from build123d import *

# Parameters (mm, degrees)
F1_DEPTH = 10.414
F2_W     = 50.8
F2_H     = 38.1
F2_R     = 17.78
F2_R_2   = 7.62
F3_DEPTH = 2.54
F4_W     = 10.16
F4_H     = 2.54
F4_R     = 1.27
F5_DEPTH = 5.08
F6_W     = 12.7
F6_H     = 2.54
F7_DEPTH = 5.08


with BuildPart() as f1:
    # F0 (on Front) → F1 (new body)
    with BuildSketch(Plane.XZ):
        with BuildLine():
            Line((-5.08, 57.662666), (-55.88, 57.662666))
            ThreePointArc((-55.88, 57.662666), (-59.472102, 56.174768), (-60.96, 52.582666))
            Line((-60.96, 52.582666), (-60.96, -41.397334))
            ThreePointArc((-60.96, -41.397334), (-59.472102, -44.989437), (-55.88, -46.477334))
            Line((-55.88, -46.477334), (-5.08, -46.477334))
            ThreePointArc((-5.08, -46.477334), (-1.487898, -44.989437), (0, -41.397334))
            Line((0, -41.397334), (0, 52.582666))
            ThreePointArc((0, 52.582666), (-1.487898, 56.174768), (-5.08, 57.662666))
        make_face()
    extrude(amount=F1_DEPTH)

    # F2 (on face) → F3 (join)
    with BuildSketch(Plane.XZ.offset(10.414)):
        with Locations((-30.48, 33.532666)):
            Rectangle(F2_W, F2_H)
        with Locations((-30.48, -15.997334)):
            Circle(F2_R)
        with Locations((-30.48, -15.997334)):
            Circle(F2_R_2, mode=Mode.SUBTRACT)
    extrude(amount=F3_DEPTH)

    # F4 (on face) → F5 (cut)
    with BuildSketch(Plane.XY.offset(57.662666)):
        with Locations((-48.26, -6.604)):
            Rectangle(F4_W, F4_H)
        with Locations((-9.593616, -6.604)):
            Circle(F4_R)
    extrude(amount=-F5_DEPTH, mode=Mode.SUBTRACT)

    # F6 (on face) → F7 (cut)
    with BuildSketch(Plane(origin=(0, 0, -46.477334), x_dir=(1, 0, 0), z_dir=(0, 0, -1))):
        with Locations((-30.48, 7.796658)):
            Rectangle(F6_W, F6_H)
    extrude(amount=-F7_DEPTH, mode=Mode.SUBTRACT)


solid = f1.part
CAD build for the part. Positions are in the model's coordinates, mm. A direction names the side the tool comes from. Give positions to 0.01 mm unless a question says otherwise; leave off trailing zeros. Loops run counter-clockwise (first coordinate to the right, second up) from the corner with the lowest first, then second, coordinate; pieces in that order, holes last. Notation, with made-up numbers: M -16.75,62 L -0.75,62 A28 cw -0.75,80 Z; hole C 52,46.25 d4. An arc over 180 degrees is marked long. Write each question's results on one line, items separated by ' | '.
Q1. Band-saw the part on A-A on z = -19.5. Write the cut outline in (x, y), and give its area (3 significant figures).
Geometry check:
outline: M -60.96,-10.41 L -47.91,-10.41 L -47.91,-12.95 L -37.25,-12.95 L -37.25,-10.41 L -23.71,-10.41 L -23.71,-12.95 L -13.05,-12.95 L -13.05,-10.41 L 0,-10.41 L 0,0 L -60.96,0 Z | area: 689 mm²
Q2. Mould opens along Z. For faces 1 (the face through (-48, -7.874, 55)), 2 (the face through (-48, -7, 52.583)), 3 (the face through (-31, -12, 14.483)), 4 (the face through (-23.441, -11.666, -18.916)) say: pulls with the +Z half, pulls with the -Z half, needs draft (parallel to the pull), parting line crosses it, or undercut.
Geometry check:
face 1: needs draft | face 2: pulls with the +Z half | face 3: undercut | face 4: undercut
Q3. Band-saw the part on D-D on z = 3. Write the cut outline in (x, y), and give its area (3 significant figures).
Geometry check:
outline: M -60.96,-10.41 L 0,-10.41 L 0,0 L -60.96,0 Z | area: 635 mm²
Q4. Band-saw the part on C-C on x = -40. Write the cut outline in (y, z).
Geometry check:
outline: M -12.95,-31.01 L -10.41,-31.01 L -10.41,-46.48 L 0,-46.48 L 0,57.66 L -10.41,57.66 L -10.41,52.58 L -12.95,52.58 L -12.95,14.48 L -10.41,14.48 L -10.41,-0.98 L -12.95,-0.98 Z
Q5. Band-saw the part on B-B on x = -30.48. Write the cut outline in (y, z), and give its area (3 significant figures).
Geometry check:
outline: M -12.95,-33.78 L -10.41,-33.78 L -10.41,-46.48 L -9.07,-46.48 L -9.07,-41.4 L -6.53,-41.4 L -6.53,-46.48 L 0,-46.48 L 0,57.66 L -10.41,57.66 L -10.41,52.58 L -12.95,52.58 L -12.95,14.48 L -10.41,14.48 L -10.41,1.78 L -12.95,1.78 L -12.95,-8.38 L -10.41,-8.38 L -10.41,-23.62 L -12.95,-23.62 Z | area: 1,220 mm²
Q6. Which spindle directions (+Z, -Z, +X, -X, +Y, -Y) get a long thin tool onto all of the face, cutting with end or side? Do faces 5 (the face through (-31, -12, 52.583)), 6 (the face through (-53.34, -7, 55)), 7 (the face through (-31, -9.067, -44)). Say none if no direction does.
Geometry check:
face 5: +Z, +X, -X, -Y | face 6: +Z | face 7: -Z
Q7. Flat gauge pins, fed straight in: P1, Ø0.8, axis at y = -6.5, z = 54.5, coming from the -X side; P2, Ø0.8, axis at x = -10, y = -7, coming from the +Z side; P3, Ø2, axis at y = -6, z = 55.5, coming from the +X side. Where does each tip first touch, or does it go through?
Geometry check:
P1: stops at x = -60.73 | P2: stops at z = 52.58 | P3: stops at x = -0.38
Q8. Probe probe 1 along Z at (x, y) = (-30.48, -11.9); probe 2 along Y at (x, z) = (-2.5, 43); probe 3 along Z at (x, y) = (-56, -2.5). List the from-to ranges inside material, lowest first.
Geometry check:
probe 1: z = -33.78 to -23.62, -8.38 to 1.78, 14.48 to 52.58 | probe 2: y = -10.41 to 0 | probe 3: z = -46.48 to 57.66
